Part model, mm, in its own coordinate system. Face numbers are marked on the shaded views. Give positions to 0.01 mm unless a question says otherwise; leave off trailing zeros. Write each loop counter-clockwise with the first axis right and the second up, starting at its lowest first coordinate (ties: lowest second). Pieces come first, ordered by that corner, then holes. Notation, with made-up numbers: (58.5, -35.75) - (83.5, -35.75) arc R18 cw to (83.5, -29.75) - close; hole circle Ø10 at (32.5, 35.5). An arc over 180 degrees is marked (long way). Answer as a JSON object with one key per item and string values. Group by question number.
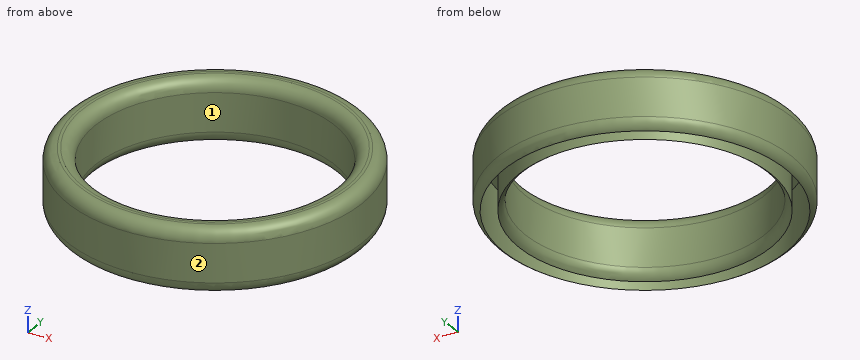
```python
from build123d import *

# Parameters (mm, degrees)
F0_R     = 59.8414566133
F0_R_2   = 48.6676693488
F3_DEPTH = 25
F7_T     = -2.5


# Not quite as in the source:
# - a fillet or chamfer that OpenCascade refuses, or shapes differently, is made with other operations: its cross-section is extruded or revolved along the edge and cut away or added
# - the program builds the solid bodies; features that only make, move or delete a surface that nothing else refers to are left out


with BuildPart() as f3:
    # F0 (on Top) → F3 (new body)
    with BuildSketch(Plane.XY):
        Circle(F0_R)
        Circle(F0_R_2, mode=Mode.SUBTRACT)
    extrude(amount=F3_DEPTH)

    # F7
    f7_openings = [f3.faces().sort_by_distance(p)[0] for p in [
        (-58.148885, 0, 0),
    ]]
    offset(amount=F7_T, openings=f7_openings)

    # F8: fillet of radius 5 on 3 edges, made by hand

    # F8_s1 → F8_t2 (revolve, cut)
    with BuildSketch(Plane.XZ):
        with BuildLine():
            ThreePointArc((59.8414566133, 4.3301270189), (59.1715836322, 1.8301270189), (57.3414566133, 0))
            Line((57.3414566133, 0), (59.8414566133, 0))
            Line((59.8414566133, 0), (59.8414566133, 4.3301270189))
        make_face()
    revolve(axis=Axis((0, 0, 0), (0, 0, 1)), mode=Mode.SUBTRACT)

    # F8_s3 → F8_t4 (revolve, cut)
    with BuildSketch(Plane.XZ):
        with BuildLine():
            ThreePointArc((59.8414566133, 20), (58.3769905192, 23.5355339059), (54.8414566133, 25))
            Line((54.8414566133, 25), (59.8414566133, 25))
            Line((59.8414566133, 25), (59.8414566133, 20))
        make_face()
    revolve(axis=Axis((0, 0, 25), (0, 0, 1)), mode=Mode.SUBTRACT)

    # F9: fillet of radius 5 on 3 edges, made by hand

    # F9_s1 → F9_t2 (revolve, cut)
    with BuildSketch(Plane.XZ):
        with BuildLine():
            ThreePointArc((48.6676693488, 4.3301270189), (49.3375423299, 1.8301270189), (51.1676693488, 0))
            Line((51.1676693488, 0), (48.6676693488, 0))
            Line((48.6676693488, 0), (48.6676693488, 4.3301270189))
        make_face()
    revolve(axis=Axis((0, 0, 0), (0, 0, 1)), mode=Mode.SUBTRACT)

    # F9_s3 → F9_t4 (revolve, cut)
    with BuildSketch(Plane.XZ):
        with BuildLine():
            ThreePointArc((53.6676693488, 25), (50.1321354429, 23.5355339059), (48.6676693488, 20))
            Line((48.6676693488, 20), (48.6676693488, 25))
            Line((48.6676693488, 25), (53.6676693488, 25))
        make_face()
    revolve(axis=Axis((0, 0, 25), (0, 0, 1)), mode=Mode.SUBTRACT)


solid = f3.part
```
1) Drop flat-ended pins along their axis: P1, Ø8, axis at x = -0.5, z = 5.5, coming from the +Y side; P2, Ø1, axis at x = -37.5, z = 9.5, coming from the +Y side; P3, Ø12, axis at y = -21, z = 4.5, coming from the -X side. Give the stop position or say it passes through.
2) Band-saw the part on A-A (z = 16). List the corners of the cut face in (x, y), plus the area to 3 significant figures.
3) Probe line 1 (Y direction, x = 0, z = 11.75); line 2 (Y direction, x = 44.5, z = 20.25); line 3 (X direction, y = 28, z = 8.5). List the from-to ranges inside material, lowest first.
4) Mould opens along X. For the marked faces 1 and 2 say: pulls with the +X half, pulls with the -X half, needs draft (parallel to the pull), parting line crosses it, or undercut.
5) Band-saw the part on B-B (y = 0). List the corners of the cut face in (x, z), plus the area to 3 significant figures.
Verdict:
{
 "1": {"P1": "y = 59.84", "P2": "y = 47.03", "P3": "x = -57.93"},
 "2": {"outline": "circle Ø119.68 at (0, 0); circle Ø102.34 at (0, 0); hole circle Ø114.68 at (0, 0); hole circle Ø97.34 at (0, 0)", "area": "1,700 mm2"},
 "3": {"line 1": "-59.84 to -57.34, -51.17 to -48.67, 48.67 to 51.17, 57.34 to 59.84", "line 2": "-40 to -36.16, -25.26 to -19.72, 19.72 to 25.26, 36.16 to 40", "line 3": "-52.89 to -50.04, -42.83 to -39.81, 39.81 to 42.83, 50.04 to 52.89"},
 "4": {"face 1": "undercut", "face 2": "parting line crosses it"},
 "5": {"outline": "(-59.84, 4.33) arc R5 ccw to (-57.34, 0) - (-57.34, 22.5) - (-51.17, 22.5) - (-51.17, 0) arc R5 ccw to (-48.67, 4.33) - (-48.67, 20) arc R5 ccw to (-53.67, 25) - (-54.84, 25) arc R5 ccw to (-59.84, 20) - close; (48.67, 4.33) arc R5 ccw to (51.17, 0) - (51.17, 22.5) - (57.34, 22.5) - (57.34, 0) arc R5 ccw to (59.84, 4.33) - (59.84, 20) arc R5 ccw to (54.84, 25) - (53.67, 25) arc R5 ccw to (48.67, 20) - close", "area": "247 mm2"}
}
